Can you work these out from the model? Positions are in its coordinate system, mm. A direction names the side the tool comes from. Round coordinates to 2 decimals unless told otherwise and drop trailing zeros. Write each loop counter-clockwise with the first axis right and the second up, starting at its lowest first coordinate (ties: lowest second). Pieces come first, ordered by that corner, then holes. Notation, with made-up numbers: (22, -16) - (29, -16) arc R30 cw to (29, 22) - close; hole circle Ø5 at (78, 43.5). An arc over 180 degrees is marked (long way). One line per item, written item: value. Start each with the question number.
(1) I'm going to push flat-ended pins straight in: pin 1 Ø1.3 at (y, z) = (4, 1.5) entering from +X; pin 2 Ø2 at (x, y) = (6, -4) entering from +Z (3 decimals); pin 3 Ø3 at (x, y) = (0, -11.43) entering from -Z; pin 4 Ø1 at (x, z) = (-9, 2) entering from +Y (3 decimals). Where does each tip first touch, or does it pass through?
(2) I want a section at A-A on z = 0.9. List the corners of the cut face in (x, y) for me (1 decimal).
(3) I want a section at B-B on y = 0. List the corners of the cut face in (x, z) for me (1 decimal).
(4) Thinking about a two-plate mould opening in X: for faces 1 (the face through (1.67, -0.53, 1.57)), 2 (the face through (5.27, -7, 2)), 3 (the face through (-5.27, 4, 2)), 4 (the face through (0, 4.762, 2)), which applies, +X half, -X half, draft (parallel to the pull), parting line (faces both ways), or undercut?
(5) I want a section at D-D on y = 3.5. List the corners of the cut face in (x, z) for me (1 decimal), plus the area to 3 significant figures.
(6) If I drill on L1, parallel to Y at x = 0, z = 1.45; L2, parallel to X at y = 0, z = 1.85; L3, parallel to X at y = -11.43, z = 0.95, over which ranges is the centre line in solid material (lowest first)? Write a range as from..to.
(7) On a 3-axis mill with a long thin cutter (end or side, diameter ignored), from which of +Z, -Z, +X, -X, +Y, -Y can I reach the whole of each face in a straight line? I mean faces 5 (the face through (-5.27, -7, 2)), 6 (the face through (-8, 3.175, 2)), 7 (the face through (8, -3.175, 2)). Say none if no direction works.
(8) I want a section at C-C on x = 0. List the corners of the cut face in (y, z) for me (1 decimal), plus the area to 3 significant figures.
from build123d import *

# Parameters (mm, degrees)
F1_DEPTH = 3.175
F2_R     = 1.7526
F3_DEPTH = 3.175
F4_R     = 1.7526
F5_DEPTH = 25.4


with BuildPart() as f1:
    # F0 (on Top) → F1 (new body)
    with BuildSketch(Plane.XY):
        Polygon((-5.2705, 3.175), (-11.1125, 3.175), (-11.1125, -3.175), (-5.2705, -3.175), (-5.2705, -4.7625), (5.2705, -4.7625), (5.2705, -3.175), (11.1125, -3.175), (11.1125, 3.175), (5.2705, 3.175), (5.2705, 4.7625), (-5.2705, 4.7625), align=None)
    extrude(amount=F1_DEPTH)

    # F2 (on face) → F3 (join, through all)
    with BuildSketch(Plane(origin=(0, 0, 0), x_dir=(1, 0, 0), z_dir=(0, 0, -1))):
        with BuildLine():
            Line((5.2705, 4.7625), (5.2705, 11.43))
            ThreePointArc((5.2705, 11.43), (0, 16.7005), (-5.2705, 11.43))
            Line((-5.2705, 11.43), (-5.2705, 4.7625))
            Line((-5.2705, 4.7625), (5.2705, 4.7625))
        make_face()
        with Locations((0, 11.43)):
            Circle(F2_R, mode=Mode.SUBTRACT)
    extrude(amount=-F3_DEPTH)

    # F4 (on face) → F5 (cut)
    with BuildSketch(Plane(origin=(0, 0, 0), x_dir=(1, 0, 0), z_dir=(0, 0, -1))):
        Circle(F4_R)
    extrude(amount=-F5_DEPTH, mode=Mode.SUBTRACT)


solid = f1.part
Established:
1. pin 1: x = 5.27
1. pin 2: z = 3.175
1. pin 3: through
1. pin 4: y = 3.175
2. outline: (-11.1, -3.2) - (-5.3, -3.2) - (-5.3, -11.4) arc R5.3 ccw to (5.3, -11.4) - (5.3, -3.2) - (11.1, -3.2) - (11.1, 3.2) - (5.3, 3.2) - (5.3, 4.8) - (-5.3, 4.8) - (-5.3, 3.2) - (-11.1, 3.2) - close; hole circle Ø3.5 at (0, -11.4); hole circle Ø3.5 at (0, 0)
3. outline: (-11.1, 0) - (-1.8, 0) - (-1.8, 3.2) - (-11.1, 3.2) - close; (1.8, 0) - (11.1, 0) - (11.1, 3.2) - (1.8, 3.2) - close
4. face 1: undercut
4. face 2: +X half
4. face 3: -X half
4. face 4: draft
5. outline: (-5.3, 0) - (5.3, 0) - (5.3, 3.2) - (-5.3, 3.2) - close
5. area: 33.5 mm2
6. L1: -16.7..-13.18, -9.68..-1.75, 1.75..4.76
6. L2: -11.11..-1.75, 1.75..11.11
6. L3: -5.27..-1.75, 1.75..5.27
7. face 5: +Z, -Z, -X, -Y
7. face 6: +Z, -Z, -X, +Y
7. face 7: +Z, -Z, +X, -Y
8. outline: (-16.7, 0) - (-13.2, 0) - (-13.2, 3.2) - (-16.7, 3.2) - close; (-9.7, 0) - (-1.8, 0) - (-1.8, 3.2) - (-9.7, 3.2) - close; (1.8, 0) - (4.8, 0) - (4.8, 3.2) - (1.8, 3.2) - close
8. area: 45.9 mm2
